CAD build for the part. Positions are in the model's coordinates, mm. A direction names the side the tool comes from. Give positions to 0.01 mm unless a question says otherwise; leave off trailing zeros. Loops run counter-clockwise (first coordinate to the right, second up) from the corner with the lowest first, then second, coordinate; pieces in that order, holes last. Notation, with made-up numbers: (84.25, 35.5) - (97.25, 35.5) arc R25 ccw to (97.25, 66.5) - close; hole circle Ø11 at (59.5, 27.5). An arc over 180 degrees is marked (long way). Return JSON: item names as keys, results as strings.
from build123d import *

# Parameters (mm, degrees)
BOSS_EXTRUDE1_DEPTH = 20
SKETCH3_R           = 4
CUT_EXTRUDE1_DEPTH  = 59.043087444
SKETCH4_R           = 3.25
CUT_EXTRUDE2_DEPTH  = 59.043087444


with BuildPart() as part:
    # Sketch1 → Boss-Extrude1 (new body)
    with BuildSketch(Plane(origin=(0, 0, 0), x_dir=(0, 0, -1), z_dir=(1, 0, 0))):
        with BuildLine():
            Line((0, 2), (0, 40))
            Line((0, 40), (3, 40))
            Line((3, 40), (3, 5))
            ThreePointArc((3, 5), (3.585786438, 3.585786438), (5, 3))
            Line((5, 3), (40, 3))
            Line((40, 3), (40, 0))
            Line((40, 0), (2, 0))
            ThreePointArc((2, 0), (0.585786438, 0.585786438), (0, 2))
        make_face()
    extrude(amount=BOSS_EXTRUDE1_DEPTH)

    # Sketch3 → Cut-Extrude1 (cut, through all)
    with BuildSketch(Plane(origin=(0, 0, -3), x_dir=(-1, 0, 0), z_dir=(0, 0, -1))):
        with Locations(Location((-10, 25, 0), (0, 0, 90))):
            Circle(SKETCH3_R)
    extrude(amount=-CUT_EXTRUDE1_DEPTH, mode=Mode.SUBTRACT)

    # Sketch4 → Cut-Extrude2 (cut, through all)
    with BuildSketch(Plane(origin=(0, 3, 0), x_dir=(1, 0, 0), z_dir=(0, 1, 0))):
        with Locations(Location((10, 32, 0), (0, 0, 270))):
            Circle(SKETCH4_R)
        with Locations(Location((10, 17, 0), (0, 0, 270))):
            Circle(SKETCH4_R)
    extrude(amount=-CUT_EXTRUDE2_DEPTH, mode=Mode.SUBTRACT)


solid = part.part
1. Cut at B-B, the plane z = -32. Write the cut outline in (x, y), plus the area to 3 significant figures.
Values follow:
{"outline": "(0, 0) - (6.75, 0) - (6.75, 3) - (0, 3) - close; (13.25, 0) - (20, 0) - (20, 3) - (13.25, 3) - close", "area": "40.5 mm²"}
2. Which spindle directions (+Z, -Z, +X, -X, +Y, -Y) get a long thin tool onto all of the face, cutting with end or side? Do faces 5 (the face through (10, 3, -22)), 6 (the face through (20, 2, -11)). Say none if no direction does.
Values follow:
{"face 5": "-Z, +X, -X, +Y", "face 6": "+Z, -Z, +X, +Y, -Y"}
3. Drop flat-ended pins along their axis: P1, Ø10, axis at x = 3.5, z = -14, coming from the -Y side; P2, Ø8.5, axis at x = 10, z = -32, coming from the +Y side; P3, Ø1.5, axis at x = 9, y = 35.5, coming from the -Z side; P4, Ø7, axis at x = 10, y = 25, coming from the -Z side. Give the stop position or say it passes through.
Values follow:
{"P1": "stops at y = 0", "P2": "stops at y = 3", "P3": "stops at z = -3", "P4": "passes through"}
4. Drill centre lines: probe 1 along X at (y, z) = (1, -32); probe 2 along Z at (x, y) = (14, 18); probe 3 along X at (y, z) = (25, -1). Where is each one in solid material? Low to high.
Values follow:
{"probe 1": "x = 0 to 6.75, 13.25 to 20", "probe 2": "z = -3 to 0", "probe 3": "x = 0 to 6, 14 to 20"}
5. Pull direction X, two halves, no side cores. Call faces 1 (the face through (10, 21, -2)), 2 (the face through (10, 40, -1)), 3 (the face through (10.143, 1.521, -20.247)), 4 (the face through (0, 2, -11)): +X half, -X half, draft (parallel to the pull), parting line (faces both ways), or undercut.
Values follow:
{"face 1": "undercut", "face 2": "draft", "face 3": "undercut", "face 4": "-X half"}
6. Cut at C-C, the plane x = 4.5. Write the cut outline in (y, z).
Values follow:
{"outline": "(0, -40) - (3, -40) - (3, -5) arc R2 cw to (5, -3) - (40, -3) - (40, 0) - (2, 0) arc R2 ccw to (0, -2) - close"}
7. Cut at D-D, the plane x = 8.25. Write the cut outline in (y, z).
Values follow:
{"outline": "(0, -40) - (3, -40) - (3, -34.74) - (0, -34.74) - close; (0, -29.26) - (3, -29.26) - (3, -19.74) - (0, -19.74) - close; (0, -14.26) - (3, -14.26) - (3, -5) arc R2 cw to (5, -3) - (21.4, -3) - (21.4, 0) - (2, 0) arc R2 ccw to (0, -2) - close; (28.6, -3) - (40, -3) - (40, 0) - (28.6, 0) - close"}
8. Cut at A-A, the plane y = 25. Write the cut outline in (x, z).
Values follow:
{"outline": "(0, -3) - (6, -3) - (6, 0) - (0, 0) - close; (14, -3) - (20, -3) - (20, 0) - (14, 0) - close"}
